```python
from build123d import *

# Parameters (mm, degrees)
SKETCH1_W           = 42
SKETCH1_H           = 60
BOSS_EXTRUDE1_DEPTH = 30
SKETCH2_R           = 10
CUT_EXTRUDE1_DEPTH  = 80.14543575
SKETCH3_R           = 2
CUT_EXTRUDE2_DEPTH  = 10


with BuildPart() as part:
    # Sketch1 → Boss-Extrude1 (new body)
    with BuildSketch(Plane(origin=(0, 0, 0), x_dir=(0, 0, -1), z_dir=(1, 0, 0))):
        with Locations((21, 30)):
            Rectangle(SKETCH1_W, SKETCH1_H)
    extrude(amount=BOSS_EXTRUDE1_DEPTH)

    # Sketch2 → Cut-Extrude1 (cut, through all)
    with BuildSketch(Plane(origin=(0, 60, 0), x_dir=(1, 0, 0), z_dir=(0, 1, 0))):
        with Locations(Location((15.5, 22.682266583, 0), (0, 0, 270))):
            Circle(SKETCH2_R)
    extrude(amount=-CUT_EXTRUDE1_DEPTH, mode=Mode.SUBTRACT)

    # Sketch3 → Cut-Extrude2 (cut)
    with BuildSketch(Plane(origin=(30, 0, 0), x_dir=(0, 0, -1), z_dir=(1, 0, 0))):
        with Locations((6, 45)):
            Circle(SKETCH3_R)
        with Locations((36, 45)):
            Circle(SKETCH3_R)
        with Locations((36, 15)):
            Circle(SKETCH3_R)
        with Locations((6, 15)):
            Circle(SKETCH3_R)
    extrude(amount=-CUT_EXTRUDE2_DEPTH, mode=Mode.SUBTRACT)


solid = part.part
```
Geometry: final body of the model. Coordinates: model frame, mm. A direction names the side the tool comes from. Round coordinates to 2 decimals unless told otherwise and drop trailing zeros. Order: outer loops, then holes, each group sorted by start corner. A loop starts at its lowest first (then second) coordinate and runs counter-clockwise, first axis right, second up. Notation, with made-up numbers: M 86.25,3 L 108.25,3 A24 cw 108.25,20 Z; hole C 87.5,-28 d4. An arc over 180 degrees is marked long. Use one line per item in the form item = value. Start each with the question number.
Q1. Cut plane A-A (y = 15). Return loops of the section in (x, z), and give its area (3 significant figures).
Q2. Cut plane B-B (x = 15.5). Return loops of the section in (y, z).
Q3. Pin query (flat end, axial travel): pin 1 Ø4.5 at (y, z) = (15, -36) entering from +X; pin 2 Ø3 at (x, z) = (11, -16.5) entering from +Y; pin 3 Ø2 at (y, z) = (45.5, -6) entering from +X. Return the tip coordinate at first contact, or that it passes through.
Q4. Cut plane D-D (x = 22.5). Return loops of the section in (y, z), and give its area (3 significant figures).
Q5. Access query for faces 1 (the face through (15, 0, -11)), 2 (the face through (25, 43, -6)). Directions: +Z, -Z, +X, -X, +Y, -Y. A direction counts if a zero-diameter tool reaches every point of the face in a straight line with its end or side. Return the directions, or none.
Q6. Cut plane C-C (z = -20). Return loops of the section in (x, y).
Q7. Material intervals for line 1 (Y direction, x = 24.75, z = -36); line 2 (X direction, y = 3.5, z = -14.5); line 3 (Z direction, x = 7.25, y = 4.5), sorted ascending. Write a range as [from, to].
Q8. Mould query, pull axis Y, two halves, no side actions, for faces 3 (the face through (30, 30, -21)), 4 (the face through (15, 60, -11)), 5 (the face through (25.07, 15.601, -37.908)). Classes: +Y half, -Y half, draft (parallel to the pull), parting line (faces both ways), or undercut.
Geometry results:
q1.outline = M 0,-42 L 30,-42 L 30,-38 L 20,-38 L 20,-34 L 30,-34 L 30,-8 L 20,-8 L 20,-4 L 30,-4 L 30,0 L 0,0 Z; hole C 15.5,-22.68 d20
q1.area = 866 mm^2
q2.outline = M 0,-42 L 60,-42 L 60,-32.68 L 0,-32.68 Z; M 0,-12.68 L 60,-12.68 L 60,0 L 0,0 Z
q3.pin_1 = 30
q3.pin_2 = through
q3.pin_3 = 20
q4.outline = M 0,-42 L 60,-42 L 60,-29.82 L 0,-29.82 Z; M 0,-15.54 L 60,-15.54 L 60,0 L 0,0 Z; hole C 15,-36 d4; hole C 15,-6 d4; hole C 45,-36 d4; hole C 45,-6 d4
q4.area = 1,610 mm^2
q5.face_1 = +Z, -Z, +X, -X, -Y
q5.face_2 = +X
q6.outline = M 0,0 L 5.87,0 L 5.87,60 L 0,60 Z; M 25.13,0 L 30,0 L 30,60 L 25.13,60 Z
q7.line_1 = [0, 13], [17, 43], [47, 60]
q7.line_2 = [0, 9.75], [21.25, 30]
q7.line_3 = [-42, -28.33], [-17.03, 0]
q8.face_3 = draft
q8.face_4 = +Y half
q8.face_5 = undercut
